Verification items for this drawing (mm, ordinates from the low corner). Coordinates: 2 decimals unless noted, no trailing zeros. Order: outer loops, then holes, each group sorted by start corner. A loop starts at its lowest first (then second) coordinate and runs counter-clockwise, first axis right, second up. Notation, with made-up numbers: (20, 50.5) - (50, 50.5) arc R20 ccw to (50, 74.5) - close; hole circle Ø9 at (-14, -10.75). An arc over 180 degrees is marked (long way). Use CSV: the item, a comma, the result in double quotes. Start each with the question number.
1) Sectioned sample at A-A, the plane y = 2.05. Record the cut outline in (x, z) (3 decimals), and give its area (3 significant figures).
2) Thickness scan on probe 1 along Z at (x, y) = (30, 0.45) (3 decimals); probe 2 along X at (y, z) = (3.05, 33) (3 decimals); probe 3 along Y at (x, z) = (58.5, 43.5) (3 decimals). Record the ranges inside material, lowest first. Write a range as [from, to].
3) Depth check by flat-ended pin: P1, Ø1, axis at x = 31.5, y = 2.5, coming from the -Z side; P2, Ø1.5, axis at y = 1, z = 42.5, coming from the +X side; P3, Ø1.5, axis at y = 1, z = 6.5, coming from the +X side; P4, Ø3, axis at x = 31.5, z = 43, coming from the -Y side. Enter the tip coordinate at first touch or a pass-through.
4) Sectioned sample at C-C, the plane x = 7.5. Record the cut outline in (y, z) (3 decimals).
5) Sectioned sample at B-B, the plane z = 23.5. Record the cut outline in (x, y) (3 decimals), and give its area (3 significant figures).
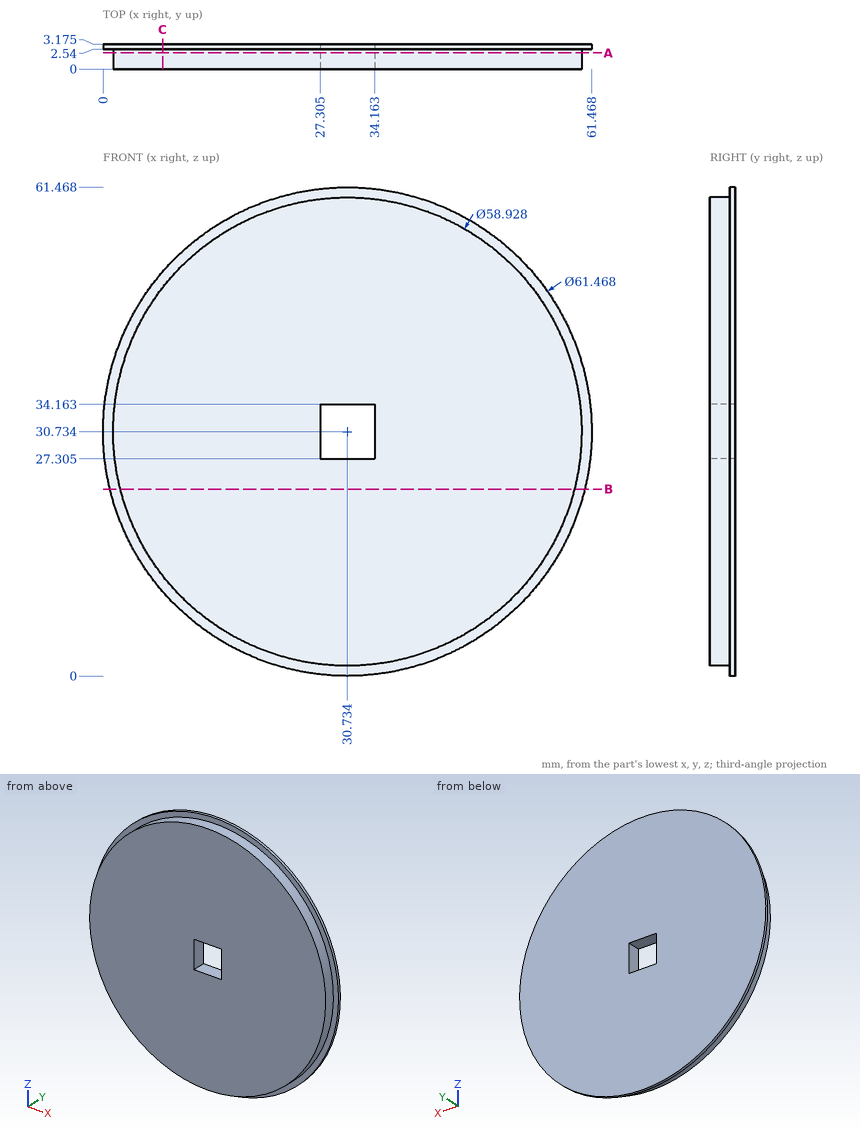
Evaluation:
1,outline,"circle Ø58.928 at (30.734, 30.734); hole (27.305, 27.305) - (34.163, 27.305) - (34.163, 34.163) - (27.305, 34.163) - close"
1,area,"2,680 mm²"
2,probe 1,"[1.279, 27.305], [34.163, 60.189]"
2,probe 2,"[0.084, 27.305], [34.163, 61.384]"
2,probe 3,"[2.54, 3.175]"
3,P1,"z = 0"
3,P2,"x = 58.06"
3,P3,"x = 48.53"
3,P4,"y = 0"
4,outline,"(0, 12.615) - (2.54, 12.615) - (2.54, 10.615) - (3.175, 10.615) - (3.175, 50.853) - (2.54, 50.853) - (2.54, 48.853) - (0, 48.853) - close"
5,outline,"(0.863, 2.54) - (2.172, 2.54) - (2.172, 0) - (59.296, 0) - (59.296, 2.54) - (60.605, 2.54) - (60.605, 3.175) - (0.863, 3.175) - close"
5,area,"183 mm²"
